Model file for the job. Use its own axes, mm. A direction names the side the tool comes from. Round coordinates to 2 decimals unless told otherwise and drop trailing zeros. Loops run counter-clockwise (first coordinate to the right, second up) from the corner with the lowest first, then second, coordinate; pieces in that order, holes last. Notation, with made-up numbers: (45.25, 49.5) - (66.25, 49.5) arc R21 cw to (66.25, 63.5) - close; hole circle Ø9 at (13.25, -22). An arc over 180 degrees is marked (long way). Use one line per item in the form item = value.
from build123d import *

# Parameters (mm, degrees)
BOSS_EXTRU_1_DEPTH      = 30
BOSS_EXTRU_2_DEPTH      = 0.5
ENL_V_MAT_EXTRU_1_DEPTH = 50
CONG_1_R                = 1.5


with BuildPart() as part:
    # Esquisse1 → Boss.-Extru.1 (new body, symmetric)
    with BuildSketch(Plane(origin=(0, 0, 0), x_dir=(0, 0, -1), z_dir=(1, 0, 0))):
        with BuildLine():
            Line((-6.318486634, -7.160951519), (6.318486634, -7.160951519))
            ThreePointArc((6.318486634, -7.160951519), (0, 9.55), (-6.318486634, -7.160951519))
        make_face()
    extrude(amount=BOSS_EXTRU_1_DEPTH, both=True)

    # Esquisse3 → Boss.-Extru.2 (add, symmetric)
    with BuildSketch(Plane(origin=(0, 0, 0), x_dir=(0, 0, -1), z_dir=(1, 0, 0))):
        with BuildLine():
            Line((-10.306467549, -7.160951519), (10.306467549, -7.160951519))
            ThreePointArc((10.306467549, -7.160951519), (0, 12.55), (-10.306467549, -7.160951519))
        make_face()
    extrude(amount=BOSS_EXTRU_2_DEPTH, both=True)

    # Esquisse2 → Enlèv. mat.-Extru.1 (cut, symmetric)
    with BuildSketch(Plane(origin=(0, 0, 0), x_dir=(0, 0, -1), z_dir=(1, 0, 0))):
        Polygon((-6.488442747, 1.194524241), (0, -5.293918507), (6.488442747, 1.194524241), (0, 7.682966988), align=None)
    extrude(amount=ENL_V_MAT_EXTRU_1_DEPTH, both=True, mode=Mode.SUBTRACT)

    # Congé1
    cong_1_edges = [part.edges().sort_by_distance(p)[0] for p in [
        (-30, 9.55, 0),
        (30, 9.55, 0),
    ]]
    fillet(cong_1_edges, radius=CONG_1_R)


solid = part.part
1. Cut at A-A, the plane x = 26. Give the cut face in (y, z).
Geometry check:
outline = (-7.16, -6.32) arc R9.55 ccw (long way) to (-7.16, 6.32) - close; hole (-5.29, 0) - (1.19, -6.49) - (7.68, 0) - (1.19, 6.49) - close
2. Pull direction Y, two halves, no side cores. Call faces 6 (the flat face through (0.42, -2.095, -3.199)), 7 (the flat face through (0.42, 4.393, -3.29)), 8 (the cylindrical face through (0.007, 12.544, -0.383)), 9 (the flat face through (0.5, 9.31, -2.73)): +Y half, -Y half, draft (parallel to the pull), parting line (faces both ways), or undercut.
Geometry check:
face_6 = undercut
face_7 = undercut
face_8 = parting line
face_9 = draft
3. Wall check: probe 1 along Z at (x, y) = (18, -1.5); probe 2 along Z at (x, y) = (-2.5, -3); probe 3 along Y at (x, z) = (16.5, 0.5). Give the ranges that are in metal, low to high.
Geometry check:
probe_1 = -9.43 to -3.79, 3.79 to 9.43
probe_2 = -9.07 to -2.29, 2.29 to 9.07
probe_3 = -7.16 to -4.79, 7.18 to 9.54
4. Flat gauge pins, fed straight in: pin 1 (10 mm diameter, centred on x = -21.5, y = -1.5, fed in from -Z); pin 2 (3 mm diameter, centred on x = 9.5, y = -4, fed in from +Z). Where does each tip first touch, or does it go through?
Geometry check:
pin_1 = -9.55
pin_2 = 9.22
5. Tool access for faces 1 (the flat face through (30, -3, 4)), 2 (the flat face through (0, -7.161, 0)), 3 (the cylindrical face through (14.696, 9.545, -0.323)), 4 (the flat face through (0.42, 4.484, 3.199)), 5 (the cylindrical face through (-14.304, 9.545, -0.323)): list every direction of +Z, -Z, +X, -X, +Y, -Y with a clear straight run to the whole face (end or side of a thin tool).
Geometry check:
face_1 = +Z, -Z, +X, +Y, -Y
face_2 = +Z, -Z, +X, -X, -Y
face_3 = +X
face_4 = +X, -X
face_5 = -X
